Design review of the part built by this model. Coordinates are the model's own, in mm. A direction names the side the tool comes from. Give positions to 0.01 mm unless a question says otherwise; leave off trailing zeros. Order: outer loops, then holes, each group sorted by start corner. A loop starts at its lowest first (then second) coordinate and runs counter-clockwise, first axis right, second up. Notation, with made-up numbers: (-33, 51) -> (3, 51) arc R17 ccw to (3, 79) -> close; hole circle Ø6 at (80, -38.75). An arc over 180 degrees is marked (long way). One line per item, written item: value. Start each with the question number.
1) Consider section D-D (z = 61). State the section outline as (x, y) points.
2) For pin 1 (1 mm diameter, centred on x = 64, z = 17, fed in from +Y); pin 2 (4 mm diameter, centred on x = 28, y = 116, fed in from -Z); pin 3 (4.5 mm diameter, centred on x = 26.5, y = 133.5, fed in from +Z); pin 4 (13.5 mm diameter, centred on x = 38.1, y = 38.1, fed in from -Z), all flat-tipped, find the tip position at first contact; note any pin that passes through.
3) Consider section A-A (z = 17.78). State the section outline as (x, y) points, plus the area to 3 significant figures.
4) Wall thickness on line 1 along Z through (x, y) = (23, 93.98); line 2 along Y through (x, z) = (38.1, 11.5); line 3 along Y through (x, z) = (12.5, 20): over which ranges is each line inside the solid? List them lowest first. Write a range as from..to.
5) Tool access review of faces 5 (the face through (38, 138, 71.12)), 6 (the face through (68.58, 129.37, 57.35)): name each direction out of +Z, -Z, +X, -X, +Y, -Y from which nothing blocks a thin tool from reaching the whole face with its end or side.
6) The part is to be moulded in two halves that separate along Z. For faces 1 (the face through (38.63, 83.83, 18.23)), 2 (the face through (29, 58, 35.56)), 3 (the face through (40.64, 9, 30)), 4 (the face through (38, 55, 0)), say which applies: released by +Z, released by -Z, zero draft, split by the parting line, or undercut.
7) Consider section B-B (x = 38.1). State the section outline as (y, z) points, plus the area to 3 significant figures.
8) Consider section C-C (y = 38.1). State the section outline as (x, z) points.
from build123d import *

# Parameters (mm, degrees)
F1_DEPTH       = 76.2
F2_R           = 10.16
F3_DEPTH       = 76.2
F5_DEPTH       = 27.94
F7_D           = 15.24
F7_CBORE_D     = 40.64
F7_CBORE_DEPTH = 10.16
F8_W           = 5.08
F8_H           = 10.16
F9_DEPTH       = 19.05


with BuildPart() as f1:
    # F0 (on Right) → F1 (new body)
    with BuildSketch(Plane.YZ):
        Polygon((0, 35.56), (0, 0), (111.76, 0), (147.32, 35.56), (147.32, 71.12), (111.76, 71.12), (93.98, 35.56), align=None)
    extrude(amount=F1_DEPTH)

    # F2 (on face) → F3 (cut, through all)
    with BuildSketch(Plane.YZ.offset(76.2)):
        with Locations((93.98, 17.78)):
            Circle(F2_R)
    extrude(amount=-F3_DEPTH, mode=Mode.SUBTRACT)

    # F4 (on face) → F5 (cut)
    with BuildSketch(Plane.XY.offset(71.12)):
        with BuildLine():
            ThreePointArc((15.24, 137.16), (7.62, 129.54), (15.24, 121.92))
            Line((15.24, 121.92), (60.96, 121.92))
            ThreePointArc((60.96, 121.92), (68.58, 129.54), (60.96, 137.16))
            Line((60.96, 137.16), (15.24, 137.16))
        make_face()
    extrude(amount=-F5_DEPTH, mode=Mode.SUBTRACT)

    # F7 (through all)
    with Locations(Plane.XY.offset(35.56)):
        with Locations((38.1, 38.1)):
            CounterBoreHole(F7_D / 2, F7_CBORE_D / 2, F7_CBORE_DEPTH)

    # F8 (on face) → F9 (cut)
    with BuildSketch(Plane.XZ):
        with Locations((38.1, 30.48)):
            Rectangle(F8_W, F8_H)
    extrude(amount=-F9_DEPTH, mode=Mode.SUBTRACT)


solid = f1.part
Checked values:
1. outline: (0, 106.7) -> (76.2, 106.7) -> (76.2, 147.32) -> (0, 147.32) -> close; hole (15.24, 121.92) -> (60.96, 121.92) arc R7.62 ccw to (60.96, 137.16) -> (15.24, 137.16) arc R7.62 ccw to start
2. pin 1: stops at y = 129.26
2. pin 2: stops at z = 2.24
2. pin 3: stops at z = 43.18
2. pin 4: passes through
3. outline: (0, 0) -> (76.2, 0) -> (76.2, 83.82) -> (0, 83.82) -> close; (0, 104.14) -> (76.2, 104.14) -> (76.2, 129.54) -> (0, 129.54) -> close; hole circle Ø15.24 at (38.1, 38.1)
3. area: 8,140 mm^2
4. line 1: z = 0..7.62, 27.94..35.56
4. line 2: y = 0..30.48, 45.72..85.99, 101.97..123.26
4. line 3: y = 0..84.07, 103.89..131.76
5. face 5: +Z, +X, -X, +Y, -Y
5. face 6: +Z
6. face 1: undercut
6. face 2: released by +Z
6. face 3: zero draft
6. face 4: released by -Z
7. outline: (0, 0) -> (30.48, 0) -> (30.48, 25.4) -> (0, 25.4) -> close; (45.72, 0) -> (111.76, 0) -> (147.32, 35.56) -> (147.32, 71.12) -> (137.16, 71.12) -> (137.16, 43.18) -> (121.92, 43.18) -> (121.92, 71.12) -> (111.76, 71.12) -> (93.98, 35.56) -> (58.42, 35.56) -> (58.42, 25.4) -> (45.72, 25.4) -> close; hole circle Ø20.32 at (93.98, 17.78)
7. area: 4,460 mm^2
8. outline: (0, 0) -> (30.48, 0) -> (30.48, 25.4) -> (17.78, 25.4) -> (17.78, 35.56) -> (0, 35.56) -> close; (45.72, 0) -> (76.2, 0) -> (76.2, 35.56) -> (58.42, 35.56) -> (58.42, 25.4) -> (45.72, 25.4) -> close
